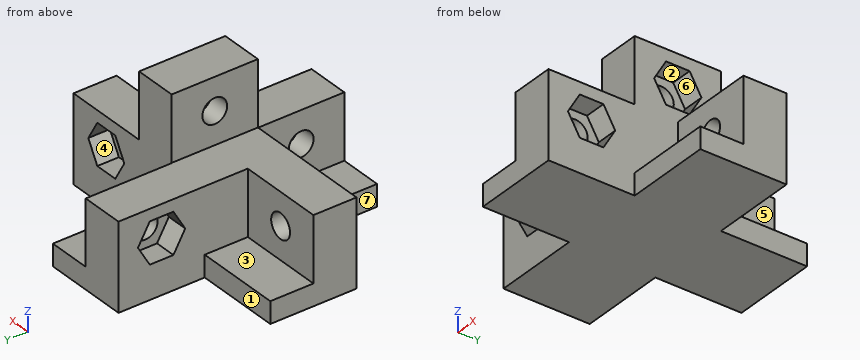
Autodesk Inventor part; units mm, degrees
ref_plane "YZ Plane" through (0, 0, 0) normal (1, 0, 0) x (0, 1, 0)
ref_plane "XZ Plane" through (0, 0, 0) normal (0, 1, 0) x (-1, 0, 0)
ref_plane "XY Plane" through (0, 0, 0) normal (0, 0, 1) x (1, 0, 0)
sketch "Sketch1" plane through (0, 0, 0) normal (0, 0, 1) x (1, 0, 0)
  line L0 (0, 0) -> (12, 0)
  line L1 (12, 0) -> (12, 12)
  line L2 (12, 12) -> (0, 12)
  line L3 (0, 12) -> (0, 0)
  line L4 (12, 12) -> (24, 12)
  line L5 (24, 12) -> (24, 0)
  line L6 (24, 0) -> (12, 0)
  line L7 (12, 0) -> (12, 12)
  line L8 (0, 0) -> (-12, 0)
  line L9 (-12, 0) -> (-12, 12)
  line L10 (-12, 12) -> (0, 12)
  line L11 (0, 12) -> (0, 0)
  line L12 (0, 0) -> (12, 0)
  line L13 (12, 0) -> (12, -12)
  line L14 (12, -12) -> (0, -12)
  line L15 (0, -12) -> (0, 0)
  line L16 (0, 12) -> (12, 12)
  line L17 (12, 12) -> (12, 24)
  line L18 (12, 24) -> (0, 24)
  line L19 (0, 24) -> (0, 12)
  dimension "d0" = 12
  dimension "d1" = 12
  dimension "d2" = 12
  dimension "d3" = 12
  dimension "d4" = 12
  dimension "d5" = 12
  dimension "d6" = 12
  dimension "d7" = 12
  dimension "d8" = 12
  dimension "d9" = 12
extrude "Extrusion1" add sketch "Sketch1" along normal blind 12
sketch "Sketch2" plane through (0, 0, 12) normal (0, 0, 1) x (1, 0, 0)
  line L0 (0, 0) -> (0, -12)
  line L1 (0, 0) -> (0, 12)
  line L2 (12, 12) -> (12, 24)
  line L3 (0, 12) -> (12, 12)
  line L4 (12, -12) -> (12, 0)
  line L5 (12, 12) -> (12, 0)
  line L6 (12, 0) -> (0, 0)
  line L7 (0, 6) -> (-12, 6)
  line L8 (-12, 12) -> (-12, 0)
  line L9 (12, 6) -> (24, 6)
  line L10 (24, 0) -> (24, 12)
  line L11 (6, 12) -> (6, 24)
  line L12 (6, 0) -> (6, -12)
  line L13 (0, -12) -> (12, -12)
  line L14 (-12, 6) -> (-12, 12)
  line L15 (0, 12) -> (-12, 12)
  line L16 (0, 12) -> (-12, 12)
  line L17 (12, 24) -> (0, 24)
  line L18 (6, 24) -> (12, 24)
  line L19 (12, 24) -> (12, 12)
  line L20 (24, 6) -> (24, 0)
  line L21 (6, -12) -> (0, -12)
  line L22 (12, 0) -> (24, 0)
extrude "Extrusion2" cut sketch "Sketch2" against normal blind 9 contours L6 L12 L13 L0 | L7 L8 L15 L1 | L5 L9 L10 L22 | L11 L17 L2 L3
sketch "Sketch3" plane through (6, 12, 12) normal (1, 0, 0) x (0, 0, -1)
  circle A0 centre (4.5, -18) radius 1.725
  line L0 (0, -24) -> (9, -24)
  line L1 (9, -24) -> (9, -12)
  point P0 (12, -12)
  dimension "d14" = 3.45
  dimension "d15" = 6
  dimension "d16" = 4.5
extrude "Extrusion3" cut sketch "Sketch3" along normal blind 3
sketch "Sketch4" plane through (12, -12, 0) normal (1, 0, 0) x (0, 0, -1)
  circle A0 centre (-7.5, 6) radius 1.725
  line L0 (-10.35, 7.6454) -> (-7.5, 9.2909)
  line L1 (-7.5, 9.2909) -> (-4.65, 7.6454)
  line L2 (-4.65, 7.6454) -> (-4.65, 4.3546)
  line L3 (-4.65, 4.3546) -> (-7.5, 2.7091)
  line L4 (-7.5, 2.7091) -> (-10.35, 4.3546)
  line L5 (-10.35, 4.3546) -> (-10.35, 7.6454)
  point P0 (0, 12)
  dimension "d19" = 2.85
extrude "Extrusion4" cut sketch "Sketch4" against normal blind 3 contours A0 | L0 L1 L2 L3 L4 L5
sketch "Sketch5" plane through (6, 12, 12) normal (1, 0, 0) x (0, 0, -1)
  circle A0 centre (4.5, 6) radius 1.725
  line L0 (12, 12) -> (0, 12)
  line L1 (0, 0) -> (0, 12)
  point P0 (12, -12)
  dimension "d22" = 3.45
  dimension "d23" = 6
  dimension "d24" = 4.5
extrude "Extrusion5" cut sketch "Sketch5" against normal blind 3
sketch "Sketch6" plane through (0, 12, 0) normal (-1, 0, 0) x (0, 0, 1)
  circle A0 centre (7.5, 6) radius 1.725
  line L0 (10.35, 4.3546) -> (7.5, 2.7091)
  line L1 (7.5, 2.7091) -> (4.65, 4.3546)
  line L2 (4.65, 4.3546) -> (4.65, 7.6454)
  line L3 (4.65, 7.6454) -> (7.5, 9.2909)
  line L4 (7.5, 9.2909) -> (10.35, 7.6454)
  line L5 (10.35, 7.6454) -> (10.35, 4.3546)
  point P0 (0, -12)
  dimension "d27" = 2.85
sketch "Sketch7" plane through (0, 0, 12) normal (0, 0, 1) x (1, 0, 0)
  line L0 (6, 12) -> (6, 24)
  line L1 (6.0413, 0) -> (6, 0)
  line L2 (6, 0) -> (6, 12)
  line L3 (6, 12) -> (6.0413, 12)
  line L4 (6.0413, 12) -> (6.0413, 0)
  line L5 (12, 0) -> (12, 6)
  line L6 (12, 0) -> (12, 12)
  line L7 (24, 12) -> (6, 12)
  line L8 (6, 0) -> (12, 0)
  point P0 (0, 0)
extrude "Extrusion6" add sketch "Sketch7" along normal blind 9 contours L4 L7 L6 L5 L8
extrude "Extrusion7" cut sketch "Sketch6" against normal blind 3 contours A0 | L0 L1 L2 L3 L4 L5
sketch "Sketch8" plane through (12, 12, 0) normal (0, 1, 0) x (1, 0, 0)
  point P0 (-12, 0)
sketch "Sketch9" plane through (12, -12, 0) normal (1, 0, 0) x (0, 0, -1)
  point P0 (0, 12)
sketch "Sketch10" plane through (12, -12, 0) normal (1, 0, 0) x (0, 0, -1)
  point P0 (0, 12)
sketch "Sketch11" plane through (6.0413, 0, 12) normal (-1, 0, 0) x (0, 0, 1)
  circle A0 centre (4.5, 6) radius 1.725
  line L0 (9, 0) -> (0, 0)
  line L1 (9, 12) -> (9, 0)
  point P0 (-12, 0)
  dimension "d32" = 3.45
  dimension "d33" = 6
  dimension "d34" = 4.5
extrude "Extrusion8" cut sketch "Sketch11" against normal blind 3
sketch "Sketch12" plane through (12, -12, 0) normal (1, 0, 0) x (0, 0, -1)
  point P0 (0, 12)
sketch "Sketch13" plane through (12, -12, 0) normal (1, 0, 0) x (0, 0, -1)
  circle A0 centre (-16.5, 18) radius 1.725
  line L0 (-19.35, 19.6454) -> (-16.5, 21.2909)
  line L1 (-16.5, 21.2909) -> (-13.65, 19.6454)
  line L2 (-13.65, 19.6454) -> (-13.65, 16.3546)
  line L3 (-13.65, 16.3546) -> (-16.5, 14.7091)
  line L4 (-16.5, 14.7091) -> (-19.35, 16.3546)
  line L5 (-19.35, 16.3546) -> (-19.35, 19.6454)
  point P0 (0, 12)
  dimension "d37" = 2.85
extrude "Extrusion9" cut sketch "Sketch13" against normal blind 3 contours A0 | L0 L1 L2 L3 L4 L5
sketch "Sketch14" plane through (12, 6, 12) normal (0, -1, 0) x (1, 0, 0)
  circle A0 centre (6, -4.5) radius 1.725
  line L0 (0, 0) -> (12, 0)
  line L1 (12, 0) -> (12, -9)
  point P0 (-12, -12)
  dimension "d40" = 3.45
  dimension "d41" = 4.5
  dimension "d42" = 6
extrude "Extrusion10" cut sketch "Sketch14" against normal blind 3
sketch "Sketch15" plane through (12, 12, 0) normal (0, 1, 0) x (1, 0, 0)
  circle A0 centre (6, -7.5) radius 1.725
  line L0 (4.3546, -10.35) -> (2.7091, -7.5)
  line L1 (2.7091, -7.5) -> (4.3546, -4.65)
  line L2 (4.3546, -4.65) -> (7.6454, -4.65)
  line L3 (7.6454, -4.65) -> (9.2909, -7.5)
  line L4 (9.2909, -7.5) -> (7.6454, -10.35)
  line L5 (7.6454, -10.35) -> (4.3546, -10.35)
  point P0 (-12, 0)
  dimension "d45" = 2.85
extrude "Extrusion11" cut sketch "Sketch15" against normal blind 3 contours A0 | L0 L1 L2 L3 L4 L5
sketch "Sketch16" plane through (-12, 6, 12) normal (0, 1, 0) x (1, 0, 0)
  circle A0 centre (6, 4.5) radius 1.725
  line L0 (12, 0) -> (0, 0)
  line L1 (0, 0) -> (0, 9)
  point P0 (12, 12)
  dimension "d48" = 3.45
  dimension "d49" = 4.5
  dimension "d50" = 6
extrude "Extrusion12" cut sketch "Sketch16" against normal blind 3
sketch "Sketch17" plane through (-12, 0, 0) normal (0, -1, 0) x (1, 0, 0)
  circle A0 centre (6, 7.5) radius 1.725
  line L0 (4.3546, 4.65) -> (2.7091, 7.5)
  line L1 (2.7091, 7.5) -> (4.3546, 10.35)
  line L2 (4.3546, 10.35) -> (7.6454, 10.35)
  line L3 (7.6454, 10.35) -> (9.2909, 7.5)
  line L4 (9.2909, 7.5) -> (7.6454, 4.65)
  line L5 (7.6454, 4.65) -> (4.3546, 4.65)
  point P0 (12, 0)
  dimension "d53" = 2.85
extrude "Extrusion13" cut sketch "Sketch17" against normal blind 3 contours A0 | L0 L1 L2 L3 L4 L5
properties part number "fourwayVer2" material "ABS Plastic"
Part model, mm, in its own coordinate system. Face numbers are marked on the shaded views. A direction names the side the tool comes from. Coordinates: 2 decimals unless noted, no trailing zeros. Order: outer loops, then holes, each group sorted by start corner. A loop starts at its lowest first (then second) coordinate and runs counter-clockwise, first axis right, second up.
(1) Slice it at A-A, the plane x = -6. Write the cut outline in (y, z) (3 decimals).
Check sheet entries:
outline: (0, 0) - (12, 0) - (12, 3) - (6, 3) - (6, 5.775) - (3, 5.775) - (3, 4.65) - (0, 4.65) - close; (0, 10.35) - (3, 10.35) - (3, 9.225) - (6, 9.225) - (6, 12) - (0, 12) - close
(2) Probe L1, parallel to Y at x = 8, z = 7.5 (3 decimals); L2, parallel to Y at x = 11, z = 17. List the from-to ranges inside material, lowest first.
Check sheet entries:
L1: y = -12 to -7.725, -4.275 to 12
L2: y = 0 to 3, 9 to 12
(3) Tool access for the marked faces 5, 6 and 7: list every direction of +Z, -Z, +X, -X, +Y, -Y with a clear straight run to the whole face (end or side of a thin tool).
Check sheet entries:
face 5: +Z, +X, +Y
face 6: +X
face 7: +Z, -Z, -X, -Y
(4) Pin check, flat tips, straight feed: pin 1 Ø3 at (y, z) = (0, 18) entering from -X; pin 2 Ø5.5 at (x, z) = (10.5, 8.5) entering from +Y; pin 3 Ø1.5 at (y, z) = (14.5, 6) entering from +X; pin 4 Ø3 at (x, z) = (19, 14.5) entering from -Y. Stop position of each tip, or through.
Check sheet entries:
pin 1: stops at x = 6.04
pin 2: stops at y = 12
pin 3: stops at x = 6
pin 4: passes through
(5) Slice it at D-D, the plane z = 3.5. Write the cut outline in (x, y).
Check sheet entries:
outline: (-12, 0) - (6, 0) - (6, -12) - (12, -12) - (12, 6) - (24, 6) - (24, 12) - (6, 12) - (6, 24) - (0, 24) - (0, 6) - (-12, 6) - close
(6) Slice it at B-B, the plane y = 1.5. Write the cut outline in (x, z).
Check sheet entries:
outline: (-12, 0) - (24, 0) - (24, 3) - (12, 3) - (12, 21) - (6.04, 21) - (6.04, 12) - (-12, 12) - close; hole (-9.29, 7.5) - (-7.65, 4.65) - (-4.35, 4.65) - (-2.71, 7.5) - (-4.35, 10.35) - (-7.65, 10.35) - close
(7) Pull direction Z, two halves, no side cores. Call the marked faces 1, 2, 3 and 4: pulls with the +Z half, pulls with the -Z half, needs draft (parallel to the pull), parting line crosses it, or undercut.
Check sheet entries:
face 1: needs draft
face 2: undercut
face 3: pulls with the +Z half
face 4: undercut
(8) Slice it at C-C, the plane y = -6. Write the cut outline in (x, z) (3 decimals).
Check sheet entries:
outline: (0, 0) - (12, 0) - (12, 4.65) - (9, 4.65) - (9, 5.775) - (6, 5.775) - (6, 3) - (0, 3) - close; (6, 9.225) - (9, 9.225) - (9, 10.35) - (12, 10.35) - (12, 12) - (6, 12) - close
